For this review, take the finished solid that the model builds, in its own axes (mm). Coordinates: 2 decimals unless noted, no trailing zeros. Write each loop counter-clockwise with the first axis right and the second up, starting at its lowest first coordinate (ties: lowest second). Pieces come first, ordered by that corner, then holes.
1) We need section A-A on z = 16.5. Write out the cut boundary in (x, y).
2) To check wall thickness, follow line 1 along X through (y, z) = (-52, 2.75); line 2 along Y through (x, z) = (390, 18.5); line 3 along X through (y, z) = (-394, 9.25). State the ranges of each line that lie inside material, in increasing order.
3) Insertion check: P1, Ø1, axis at x = -125, z = 22.5, coming from the -Y side; P2, Ø6, axis at x = 211.5, z = 20.5, coming from the -Y side; P3, Ø10, axis at y = -276, z = 8.5, coming from the +X side. Each pin has a flat end and moves straight along its axis. Give the tip position at first contact, or say it passes through.
from build123d import *

# Parameters (mm, degrees)
F1_DEPTH = 25.4
F2_R     = 5.08
F3_R     = 5.08
F4_R     = 5.08
F5_R     = 5.08
F6_R     = 5.08
F9_R     = 5.08
F10_R    = 5.08


# Not quite as in the source:
# - the program builds the solid bodies; features that only make, move or delete a surface that nothing else refers to are left out


with BuildPart() as f1:
    # F0 (on Top) → F1 (new body)
    with BuildSketch(Plane.XY):
        with BuildLine():
            Line((596.8167068857, 124.9892751187), (596.8167068857, 724.9880751187))
            Line((596.8167068857, 724.9880751187), (-603.1832931143, 724.9880751187))
            Line((-603.1832931143, 724.9880751187), (-603.1832931143, -475.0095248813))
            Line((-603.1832931143, -475.0095248813), (-3.1820931143, -475.0095248813))
            ThreePointArc((-3.1820931143, -475.0095248813), (172.5534867019, -50.7463046975), (596.8167068857, 124.9892751187))
        make_face()
    extrude(amount=F1_DEPTH)

    # F2
    f2_edges = [f1.edges().sort_by_distance(p)[0] for p in [
        (-603.183293, -475.009525, 12.7),
    ]]
    fillet(f2_edges, radius=F2_R)

    # F3
    f3_edges = [f1.edges().sort_by_distance(p)[0] for p in [
        (-3.182093, -475.009525, 12.7),
    ]]
    fillet(f3_edges, radius=F3_R)

    # F4
    f4_edges = [f1.edges().sort_by_distance(p)[0] for p in [
        (596.816707, 124.989275, 12.7),
    ]]
    fillet(f4_edges, radius=F4_R)

    # F5
    f5_edges = [f1.edges().sort_by_distance(p)[0] for p in [
        (596.816707, 724.988075, 12.7),
    ]]
    fillet(f5_edges, radius=F5_R)

    # F6
    f6_edges = [f1.edges().sort_by_distance(p)[0] for p in [
        (-603.183293, 724.988075, 12.7),
    ]]
    fillet(f6_edges, radius=F6_R)

    # F9
    f9_edges = [f1.edges().sort_by_distance(p)[0] for p in [
        (-303.172031, -475.009525, 0),
    ]]
    fillet(f9_edges, radius=F9_R)

    # F10
    f10_edges = [f1.edges().sort_by_distance(p)[0] for p in [
        (-303.172031, -475.009525, 25.4),
    ]]
    fillet(f10_edges, radius=F10_R)


solid = f1.part
Result:
1. outline: (-603.18, -469.93) arc R5.08 ccw to (-598.1, -475.01) - (-8.24, -475.01) arc R5.08 ccw to (-3.16, -469.97) arc R600 cw to (591.78, 124.97) arc R5.08 ccw to (596.82, 130.05) - (596.82, 719.91) arc R5.08 ccw to (591.74, 724.99) - (-598.1, 724.99) arc R5.08 ccw to (-603.18, 719.91) - close
2. line 1: x = -602.62 to 170.51
2. line 2: y = 88.22 to 724.99
2. line 3: x = -603.18 to 2.31
3. P1: stops at y = -474.72
3. P2: stops at y = -17.61
3. P3: stops at x = 32.57
